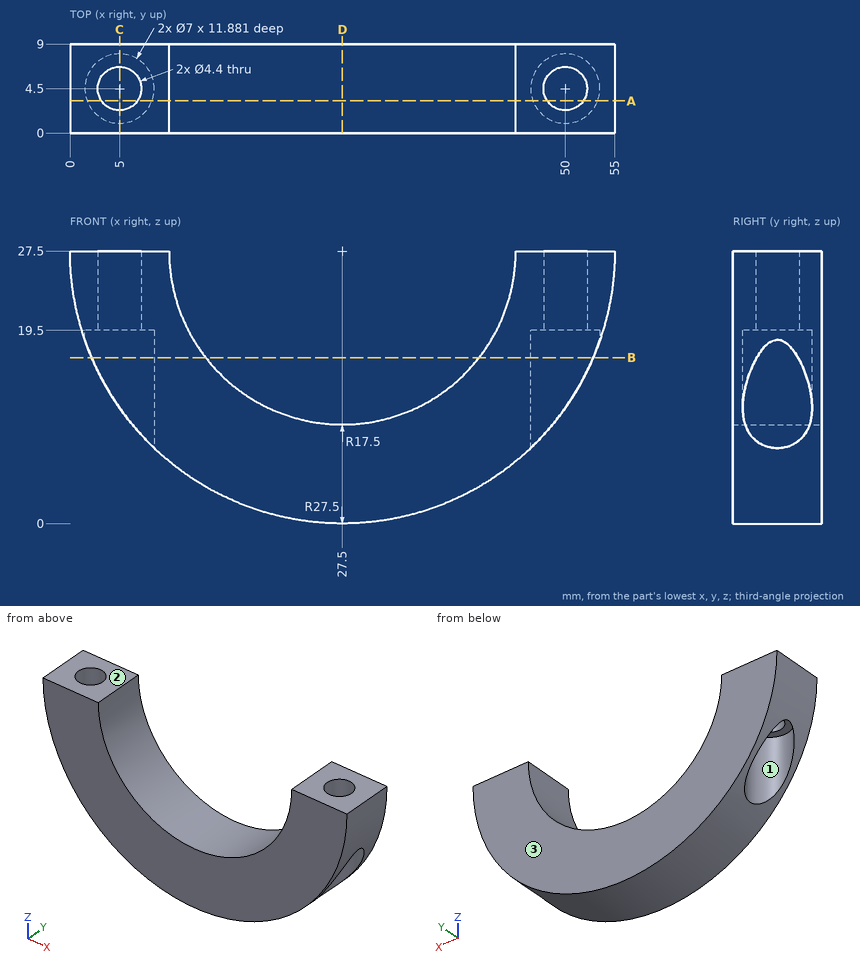
Source: three-view drawing plus pictorial views. Frame: mm from the lowest corner of the part. Coordinates: 2 decimals unless noted, no trailing zeros. Order: outer loops, then holes, each group sorted by start corner. A loop starts at its lowest first (then second) coordinate and runs counter-clockwise, first axis right, second up. Notation, with made-up numbers: M 19.25,-19.5 L 30.25,-19.5 A26 cw 30.25,8.5 Z; hole C 64.5,68.25 d9. An arc over 180 degrees is marked long. One line per question, with ' | ' between items.
Item 1: Section B-B (z = 16.75). Output: boundary loops of the cut face in (x, y), then the cut area to 3 significant figures.
Geometry results:
outline: M 2.19,0 L 13.69,0 L 13.69,9 L 2.19,9 L 2.19,6.58 A3.5 cw long 2.19,2.42 Z; M 41.31,0 L 52.81,0 L 52.81,2.42 A3.5 cw long 52.81,6.58 L 52.81,9 L 41.31,9 Z | area: 134 mm^2
Item 2: Section A-A (y = 3.25). Output: boundary loops of the cut face in (x, z).
Geometry results:
outline: M 0,27.5 A27.5 ccw 1.73,17.9 L 1.73,19.5 L 3.19,19.5 L 3.19,27.5 Z; M 6.81,19.5 L 8.27,19.5 L 8.27,7.84 A27.5 ccw 46.73,7.84 L 46.73,19.5 L 48.19,19.5 L 48.19,27.5 L 45,27.5 A17.5 cw 10,27.5 L 6.81,27.5 Z; M 51.81,19.5 L 53.27,19.5 L 53.27,17.9 A27.5 ccw 55,27.5 L 51.81,27.5 Z
Item 3: Ray query, line 1 along Y through (x, z) = (5, 12.5); line 2 along X through (y, z) = (4, 21); line 3 along Y through (x, z) = (5, 23.25). Return the intervals inside material, ascending.
Geometry results:
line 1: y = 0 to 1, 8 to 9 | line 2: x = 0.78 to 2.86, 7.14 to 11.25, 43.75 to 47.86, 52.14 to 54.22 | line 3: y = 0 to 2.3, 6.7 to 9
Item 4: Section C-C (x = 5). Output: boundary loops of the cut face in (y, z).
Geometry results:
outline: M 0,11.69 L 1,11.69 L 1,19.5 L 2.3,19.5 L 2.3,27.5 L 0,27.5 Z; M 6.7,19.5 L 8,19.5 L 8,11.69 L 9,11.69 L 9,27.5 L 6.7,27.5 Z
Item 5: Pin query (flat end, axial travel): pin 1 (3.5 mm diameter, centred on x = 49.5, y = 5, fed in from -Z); pin 2 (5 mm diameter, centred on x = 34.5, y = 1.5, fed in from +Z); pin 3 (4 mm diameter, centred on x = 50, y = 4.5, fed in from +Z); pin 4 (5 mm diameter, centred on x = 32, y = 2, fed in from +Z). Return the tip coordinate at first contact, or that it passes through.
Geometry results:
pin 1: stops at z = 19.5 | pin 2: stops at z = 12.8 | pin 3: passes through | pin 4: stops at z = 11.46
Item 6: Section D-D (x = 27.5). Output: boundary loops of the cut face in (y, z).
Geometry results:
outline: M 0,0 L 9,0 L 9,10 L 0,10 Z
Item 7: Draft query along Y for the marked faces 1, 2 and 3. Return one class per face: released by +Y, released by -Y, zero draft, split by the parting line, or undercut.
Geometry results:
face 1: undercut | face 2: zero draft | face 3: released by +Y
